The model under review builds one solid part; all positions refer to its coordinate system, in mm. Face numbers are marked on the shaded views. Coordinates: 2 decimals unless noted, no trailing zeros. Loops run counter-clockwise (first coordinate to the right, second up) from the corner with the lowest first, then second, coordinate; pieces in that order, holes last. Notation, with made-up numbers: M -14.5,45 L 34.5,45 A8 ccw 34.5,49 Z; hole C 10,67.25 d3. An arc over 180 degrees is marked long. One line per item, written item: value.
```python
from build123d import *

# Parameters (mm, degrees)
F0_W     = 450
F0_H     = 450
F1_DEPTH = 950
F2_W     = 50
F2_H     = 50
F2_W_2   = 330
F2_H_2   = 425
F3_DEPTH = 450.001
F4_W     = 380
F4_H     = 425
F5_DEPTH = 450.001
F6_W     = 373.3073347807
F6_H     = 50
F6_H_2   = 302.6243293636
F7_DEPTH = 134.2592361444


with BuildPart() as f1:
    # F0 (on Top) → F1 (new body)
    with BuildSketch(Plane.XY):
        Rectangle(F0_W, F0_H)
    extrude(amount=F1_DEPTH)

    # F2 (on face) → F3 (cut, through all)
    with BuildSketch(Plane.XZ.offset(225)):
        with Locations((200, 450)):
            Rectangle(F2_W, F2_H)
        Polygon((-225, 475), (140, 475), (190, 950), (-225, 950), align=None)
        Polygon((175, 475), (225, 475), (225, 950), align=None)
        with Locations((-25, 212.5)):
            Rectangle(F2_W_2, F2_H_2)
        with Locations((200, 212.5)):
            Rectangle(F2_W, F2_H_2)
    extrude(amount=-F3_DEPTH, mode=Mode.SUBTRACT)

    # F4 (on face) → F5 (cut, through all)
    with BuildSketch(Plane(origin=(-225, 0, 0), x_dir=(0, -1, 0), z_dir=(-1, 0, 0))):
        with Locations((0, 212.5)):
            Rectangle(F4_W, F4_H)
    extrude(amount=-F5_DEPTH, mode=Mode.SUBTRACT)

    # F6 (on face) → F7 (cut, through all)
    with BuildSketch(Plane(origin=(89.0136986301, 0, -9.3698630137), x_dir=(0, -1, 0), z_dir=(-0.9945054529, 0, 0.1046847845))):
        with Locations((3.3463326097, 864.6702893338)):
            Rectangle(F6_W, F6_H)
        with Locations((3.3463326097, 638.358124652)):
            Rectangle(F6_W, F6_H_2)
    extrude(amount=-F7_DEPTH, mode=Mode.SUBTRACT)


solid = f1.part
```
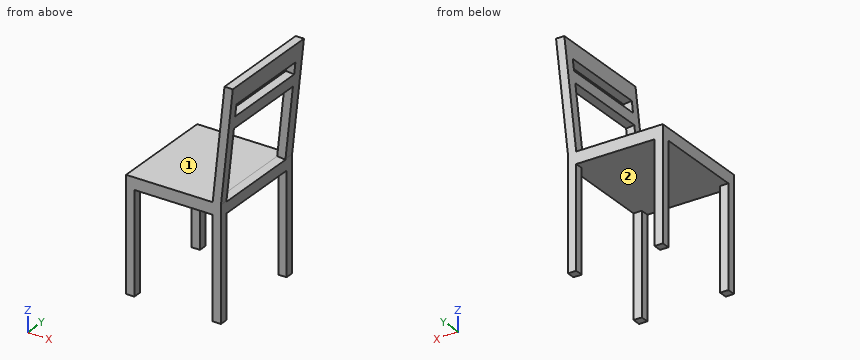
(1) Add section A-A on y = 38. State the section outline as (x, z) points, then the cut area to 3 significant figures.
Checks:
outline: M -225,425 L 175,425 L 175,471.32 L 140,475 L -225,475 Z; M 171.68,775.96 L 206.3,772.32 L 211.53,822.04 L 176.91,825.69 Z; M 182.15,875.41 L 216.77,871.77 L 225,950 L 190,950 Z
area: 24,400 mm^2
(2) Insertion check: pin 1 Ø2 at (x, y) = (-73, 128) entering from -Z; pin 2 Ø10.5 at (y, z) = (203.5, 192) entering from +X; pin 3 Ø2 at (y, z) = (11, 816.5) entering from -X. Each pin has a flat end and moves straight along its axis. Give the tip position at first contact, or say it passes through.
Checks:
pin 1: z = 425
pin 2: x = 175
pin 3: x = 175.84
(3) Add section C-C on z = 759. State the section outline as (x, y) points.
Checks:
outline: M 169.89,-225 L 204.89,-225 L 204.89,-190 L 169.89,-190 Z; M 169.89,183.31 L 204.89,183.31 L 204.89,225 L 169.89,225 Z
(4) Add section B-B on z = 141. State the section outline as (x, y) points.
Checks:
outline: M -225,-225 L -190,-225 L -190,-190 L -225,-190 Z; M -225,190 L -190,190 L -190,225 L -225,225 Z; M 140,-225 L 175,-225 L 175,-190 L 140,-190 Z; M 140,190 L 175,190 L 175,225 L 140,225 Z
(5) Add section D-D on x = -138.5. State the section outline as (y, z) points.
Checks:
outline: M -225,425 L 225,425 L 225,475 L -225,475 Z
(6) Draft analysis for pull direction X (two halves, no side actions). For the marked faces 1 and 2, state which applies: pulls with the +X half, pulls with the -X half, needs draft (parallel to the pull), parting line crosses it, or undercut.
Checks:
face 1: needs draft
face 2: undercut
(7) To check wall thickness, follow L1, parallel to Y at x = 174, z = 167; L2, parallel to Z at x = -13, y = 17.5; L3, parallel to Z at x = 192, y = 113.5. State the ranges of each line that lie inside material, in increasing order. Write a range as [from, to].
Checks:
L1: [-225, -190], [190, 225]
L2: [425, 475]
L3: [773.82, 824.1], [874.38, 950]
